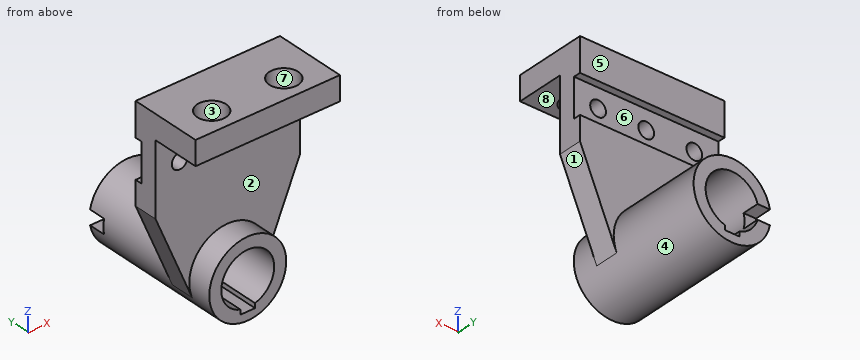
from build123d import *

# Parameters (mm, degrees)
BOSS_EXTRUDE1_DEPTH      = 10
SKETCH3_W                = 60
SKETCH3_H                = 10
BOSS_EXTRUDE2_DEPTH      = 20
SKETCH4_R                = 6
CUT_EXTRUDE1_DEPTH       = 20
SKETCH5_W                = 60
SKETCH5_H                = 16
CUT_EXTRUDE2_DEPTH       = 3
SKETCH6_R                = 3.270829893
CUT_EXTRUDE3_DEPTH       = 20
BOSS_EXTRUDE4_DEPTH      = 40
BOSS_EXTRUDE4_DEPTH_BACK = 20
SKETCH7_R                = 16
SKETCH10_W               = 12.846934043
SKETCH10_H               = 6
CUT_EXTRUDE4_DEPTH       = 7


with BuildPart() as part:
    # Sketch2 → Boss-Extrude1 (new body)
    with BuildSketch(Plane(origin=(0, 0, 0), x_dir=(1, 0, 0), z_dir=(0, 1, 0))):
        with BuildLine():
            Line((-26.355501721, -12.852372891), (33.644498279, -12.852372891))
            Line((33.644498279, -12.852372891), (33.644498279, 27.147627109))
            Line((33.644498279, 27.147627109), (18.389502388, 63.359297885))
            ThreePointArc((18.389502388, 63.359297885), (3.644498279, 73.147627109), (-11.10050583, 63.359297885))
            Line((-11.10050583, 63.359297885), (-26.355501721, 27.147627109))
            Line((-26.355501721, 27.147627109), (-26.355501721, -12.852372891))
        make_face()
        with BuildLine():
            Line((0.644498279, 69.647627109), (6.644498279, 69.647627109))
            Line((6.644498279, 69.647627109), (6.644498279, 67.730632354))
            ThreePointArc((6.644498279, 67.730632354), (3.644498279, 46.147627109), (0.644498279, 67.730632354))
            Line((0.644498279, 67.730632354), (0.644498279, 69.647627109))
        make_face(mode=Mode.SUBTRACT)
    extrude(amount=BOSS_EXTRUDE1_DEPTH)

    # Sketch3 → Boss-Extrude2 (add)
    with BuildSketch(Plane.XZ):
        with Locations((3.644498279, 7.852372891)):
            Rectangle(SKETCH3_W, SKETCH3_H)
    extrude(amount=BOSS_EXTRUDE2_DEPTH)

    # Sketch4 → Cut-Extrude1 (cut)
    with BuildSketch(Plane.XY.offset(12.852372891)):
        with Locations((-11.355501721, -10)):
            Circle(SKETCH4_R)
        with Locations((18.644498279, -10)):
            Circle(SKETCH4_R)
    extrude(amount=-CUT_EXTRUDE1_DEPTH, mode=Mode.SUBTRACT)

    # Sketch5 → Cut-Extrude2 (cut)
    with BuildSketch(Plane(origin=(0, 10, 0), x_dir=(1, 0, 0), z_dir=(0, 1, 0))):
        with Locations((3.644498279, 9.147627109)):
            Rectangle(SKETCH5_W, SKETCH5_H)
    extrude(amount=-CUT_EXTRUDE2_DEPTH, mode=Mode.SUBTRACT)

    # Sketch6 → Cut-Extrude3 (cut)
    with BuildSketch(Plane(origin=(0, 7, 0), x_dir=(1, 0, 0), z_dir=(0, 1, 0))):
        with Locations(Location((-16.355501721, 9.147627109, 0), (0, 0, 270))):
            Circle(SKETCH6_R)
        with Locations(Location((3.644498279, 9.147627109, 0), (0, 0, 270))):
            Circle(SKETCH6_R)
        with Locations(Location((23.644498279, 9.147627109, 0), (0, 0, 270))):
            Circle(SKETCH6_R)
    extrude(amount=-CUT_EXTRUDE3_DEPTH, mode=Mode.SUBTRACT)

    # Sketch7 → Boss-Extrude4 (add, two sides: drawn at the far end of the back side and taken through both)
    with BuildSketch(Plane(origin=(0, 10, 0), x_dir=(1, 0, 0), z_dir=(0, 1, 0)).offset(-BOSS_EXTRUDE4_DEPTH_BACK)):
        with Locations(Location((3.644498279, 57.147627109, 0), (0, 0, 270))):
            Circle(SKETCH7_R)
        with BuildLine():
            Line((6.644498279, 67.730632354), (6.644498279, 69.647627109))
            Line((6.644498279, 69.647627109), (0.644498279, 69.647627109))
            Line((0.644498279, 69.647627109), (0.644498279, 67.730632354))
            ThreePointArc((0.644498279, 67.730632354), (3.644498279, 46.147627109), (6.644498279, 67.730632354))
        make_face(mode=Mode.SUBTRACT)
    extrude(amount=BOSS_EXTRUDE4_DEPTH + BOSS_EXTRUDE4_DEPTH_BACK)

    # Sketch10 → Cut-Extrude4 (cut)
    with BuildSketch(Plane(origin=(0, 50, 0), x_dir=(1, 0, 0), z_dir=(0, 1, 0))):
        with Locations((-7.355501722, 57.147627109)):
            Rectangle(SKETCH10_W, SKETCH10_H)
    extrude(amount=-CUT_EXTRUDE4_DEPTH, mode=Mode.SUBTRACT)


solid = part.part
The model under review builds one solid part; all positions refer to its coordinate system, in mm. Face numbers are marked on the shaded views. A direction names the side the tool comes from. Round coordinates to 2 decimals unless told otherwise and drop trailing zeros. Loops run counter-clockwise (first coordinate to the right, second up) from the corner with the lowest first, then second, coordinate; pieces in that order, holes last. Notation, with made-up numbers: (12.5, 43.25) -> (70.5, 43.25) arc R8 cw to (70.5, 53.25) -> close; hole circle Ø2 at (86, -28.5). An arc over 180 degrees is marked (long way). Answer as CSV lines item,"result".
1) Add section D-D on y = -14. Write out the cut boundary in (x, z), plus the area to 3 significant figures.
Geometry results:
outline,"(-26.36, 2.85) -> (-15.83, 2.85) -> (-15.83, 12.85) -> (-26.36, 12.85) -> close; (-6.88, 2.85) -> (14.17, 2.85) -> (14.17, 12.85) -> (-6.88, 12.85) -> close; (23.12, 2.85) -> (33.64, 2.85) -> (33.64, 12.85) -> (23.12, 12.85) -> close"
area,"421 mm²"
2) Add section A-A on y = 8.5. Write out the cut boundary in (x, z), plus the area to 3 significant figures.
Geometry results:
outline,"(-26.36, -27.15) -> (-11.1, -63.36) arc R16 ccw to (18.39, -63.36) -> (33.64, -27.15) -> (33.64, -17.15) -> (-26.36, -17.15) -> close; (-26.36, -1.15) -> (33.64, -1.15) -> (33.64, 12.85) -> (-26.36, 12.85) -> close; hole (0.64, -69.65) -> (6.64, -69.65) -> (6.64, -67.73) arc R11 ccw (long way) to (0.64, -67.73) -> close"
area,"2,880 mm²"
3) For P1, Ø8.5, axis at x = 23.64, z = -9.15, coming from the +Y side; P2, Ø5.5, axis at x = -8.5, y = 47.5, coming from the +Z side; P3, Ø2, axis at x = -0.5, y = 22, coming from the -Z side; P4, Ø8, axis at x = 21, y = -9.5, coming from the +Z side, all flat-tipped, find the tip position at first contact; note any pin that passes through.
Geometry results:
P1,"stops at y = 7"
P2,"stops at z = -44.2"
P3,"stops at z = -72.84"
P4,"stops at z = 12.85"
4) Add section B-B on x = -8.5. Write out the cut boundary in (y, z).
Geometry results:
outline,"(-20, 2.85) -> (-15.28, 2.85) -> (-15.28, 12.85) -> (-20, 12.85) -> close; (-10, -67.56) -> (50, -67.56) -> (50, -60.15) -> (43, -60.15) -> (43, -54.15) -> (50, -54.15) -> (50, -46.73) -> (10, -46.73) -> (10, -17.15) -> (7, -17.15) -> (7, -1.15) -> (10, -1.15) -> (10, 12.85) -> (-4.72, 12.85) -> (-4.72, 2.85) -> (0, 2.85) -> (0, -46.73) -> (-10, -46.73) -> close"
5) To check wall thickness, follow line 1 along Z through (x, y) = (4, 2); line 2 along Z through (x, y) = (3.5, 19.5); line 3 along Z through (x, y) = (8.5, -7). State the ranges of each line that lie inside material, in increasing order. Write a range as from..to.
Geometry results:
line 1,"z = -73.14..-69.65, -46.15..-12.4, -5.9..12.85"
line 2,"z = -73.15..-69.65, -46.15..-41.15"
line 3,"z = -72.39..-67.02, -47.28..-41.9, 2.85..12.85"
6) Tool access review of the marked faces 4, 5, 6, 7 and 8: name each direction out of +Z, -Z, +X, -X, +Y, -Y from which nothing blocks a thin tool from reaching the whole face with its end or side.
Geometry results:
face 4,"none"
face 5,"+Z, +X, -X, +Y"
face 6,"+X, -X, +Y"
face 7,"+Z"
face 8,"+X, -X, -Y"
7) Add section C-C on z = -48.5. Write out the cut boundary in (x, y).
Geometry results:
outline,"(-17.36, 0) -> (-9.82, 0) -> (-9.82, -10) -> (-3.15, -10) -> (-3.15, 50) -> (-9.82, 50) -> (-9.82, 10) -> (-17.36, 10) -> close; (10.44, -10) -> (17.11, -10) -> (17.11, 0) -> (24.65, 0) -> (24.65, 10) -> (17.11, 10) -> (17.11, 50) -> (10.44, 50) -> close"
8) Draft analysis for pull direction Y (two halves, no side actions). For the marked faces 1, 2 and 3, state which applies: pulls with the +Y half, pulls with the -Y half, needs draft (parallel to the pull), parting line crosses it, or undercut.
Geometry results:
face 1,"needs draft"
face 2,"pulls with the -Y half"
face 3,"undercut"
